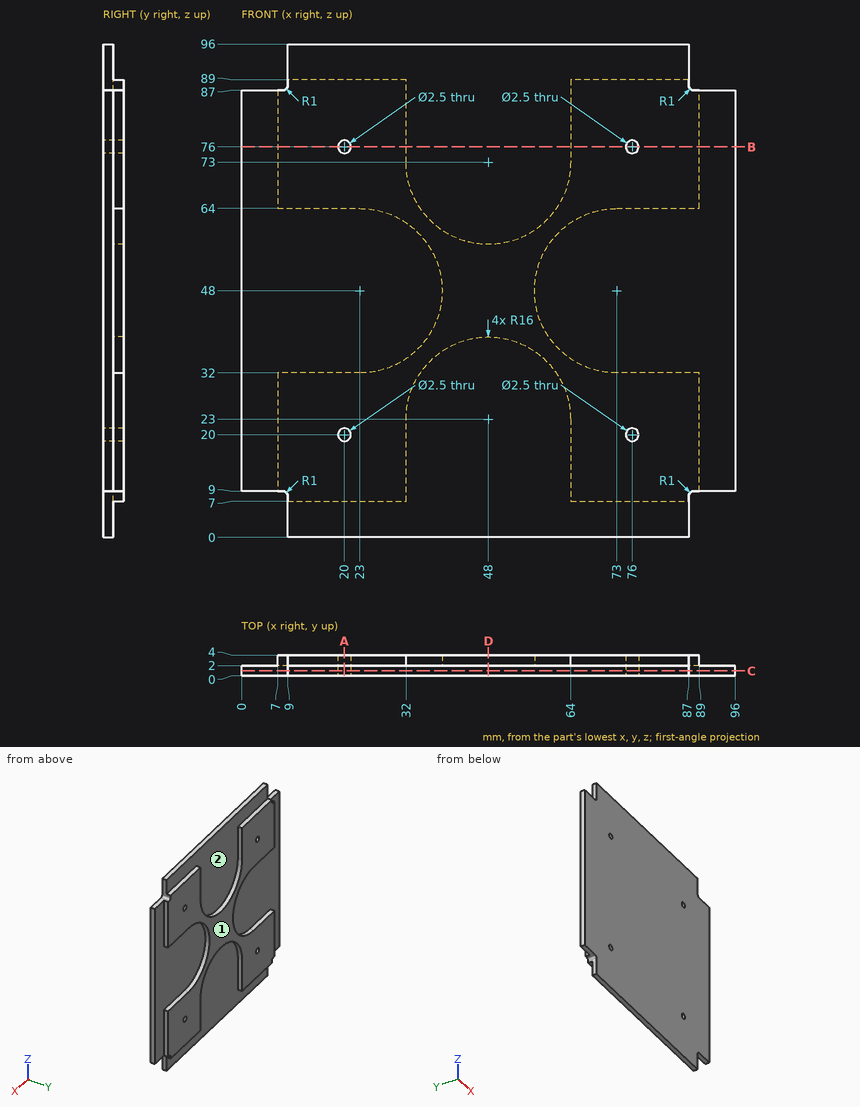
The figure shows three views and two pictorial views of one solid part (mm, origin at its lowest corner). Answer the questions. Coordinates: 2 decimals unless noted, no trailing zeros. Write each loop counter-clockwise with the first axis right and the second up, starting at its lowest first coordinate (ties: lowest second). Pieces come first, ordered by that corner, then holes. Notation, with made-up numbers: (-7, -5) -> (15, -5) arc R24 cw to (15, 23) -> close; hole circle Ø4 at (20, -29). An arc over 180 degrees is marked (long way). Return JSON: item names as keys, results as strings.
1. Determine the mould class of the marked faces 1 and 2 for opening direction X: pulls with the +X half, pulls with the -X half, needs draft (parallel to the pull), parting line crosses it, or undercut.
Found:
{"face 1": "needs draft", "face 2": "undercut"}
2. Each of these flat-tipped pins is pushed along its axis until it touches: P1, Ø2, axis at y = 1.5, z = 5, coming from the -X side; P2, Ø1.6, axis at y = 3, z = 76, coming from the +X side; P3, Ø2, axis at x = 24, y = 3.5, coming from the +Z side; P4, Ø2, axis at x = 76, z = 20, coming from the -Y side. Where does it stop, or does it pass through?
Found:
{"P1": "x = 9", "P2": "x = 89", "P3": "z = 89", "P4": "through"}
3. A cutting plane is placed at A-A (x = 20). Determine the outline of the cut face in (y, z).
Found:
{"outline": "(0, 0) -> (2, 0) -> (2, 7) -> (4, 7) -> (4, 18.75) -> (0, 18.75) -> close; (0, 21.25) -> (4, 21.25) -> (4, 32) -> (2, 32) -> (2, 64) -> (4, 64) -> (4, 74.75) -> (0, 74.75) -> close; (0, 77.25) -> (4, 77.25) -> (4, 89) -> (2, 89) -> (2, 96) -> (0, 96) -> close"}
4. A cutting plane is placed at D-D (x = 48). Determine the outline of the cut face in (y, z), and give its area (3 significant figures).
Found:
{"outline": "(0, 0) -> (2, 0) -> (2, 39) -> (4, 39) -> (4, 57) -> (2, 57) -> (2, 96) -> (0, 96) -> close", "area": "228 mm2"}
5. Find the intervals of material crossed by line 1 along X through (y, z) = (2.1, 76); line 2 along Z through (x, y) = (76, 1.5), in increasing order. Write a range as from..to.
Found:
{"line 1": "7..18.75, 21.25..32, 64..74.75, 77.25..89", "line 2": "0..18.75, 21.25..74.75, 77.25..96"}
6. A cutting plane is placed at B-B (z = 76). Determine the outline of the cut face in (x, y), and give its area (3 significant figures).
Found:
{"outline": "(0, 0) -> (18.75, 0) -> (18.75, 4) -> (7, 4) -> (7, 2) -> (0, 2) -> close; (21.25, 0) -> (74.75, 0) -> (74.75, 4) -> (64, 4) -> (64, 2) -> (32, 2) -> (32, 4) -> (21.25, 4) -> close; (77.25, 0) -> (96, 0) -> (96, 2) -> (89, 2) -> (89, 4) -> (77.25, 4) -> close", "area": "272 mm2"}
7. A cutting plane is placed at C-C (y = 1). Determine the outline of the cut face in (x, z), and give its area (3 significant figures).
Found:
{"outline": "(0, 9) -> (8, 9) arc R1 cw to (9, 8) -> (9, 0) -> (87, 0) -> (87, 8) arc R1 cw to (88, 9) -> (96, 9) -> (96, 87) -> (88, 87) arc R1 cw to (87, 88) -> (87, 96) -> (9, 96) -> (9, 88) arc R1 cw to (8, 87) -> (0, 87) -> close; hole circle Ø2.5 at (20, 20); hole circle Ø2.5 at (20, 76); hole circle Ø2.5 at (76, 20); hole circle Ø2.5 at (76, 76)", "area": "8,870 mm2"}
